Source: CAD feature listing. Evaluate the final solid. Frame: model axes, mm. A direction names the side the tool comes from. Round coordinates to 2 decimals unless told otherwise and drop trailing zeros. Loops run counter-clockwise (first coordinate to the right, second up) from the corner with the lowest first, then second, coordinate; pieces in that order, holes last. Notation, with made-up numbers: M 24.25,49.5 L 48.25,49.5 A20 cw 48.25,85.5 Z; hole C 64.25,60 d6. An arc over 180 degrees is marked long. Answer as a JSON object with one key per item and string values.
from build123d import *

# Parameters (mm, degrees)
F0_W      = 76.2
F0_H      = 38.1
F1_DEPTH  = 12.7
F2_W      = 14.097
F2_H      = 38.1
F3_DEPTH  = 0.762
F4_W      = 15.113
F4_H      = 3.048
F4_W_2    = 30.226
F5_DEPTH  = 38.101
F6_R      = 9.525
F7_DEPTH  = 6.35
F8_R      = 2.7813
F9_DEPTH  = 3.303
F10_R     = 3.3782
F11_DEPTH = 12.701
F12_R     = 0.762


with BuildPart() as f1:
    # F0 (on Top) → F1 (new body)
    with BuildSketch(Plane.XY):
        with Locations((38.1, -19.05)):
            Rectangle(F0_W, F0_H)
    extrude(amount=-F1_DEPTH)

    # F2 (on face) → F3 (cut)
    with BuildSketch(Plane.XY):
        with Locations((38.1127, -19.05)):
            Rectangle(F2_W, F2_H)
    extrude(amount=-F3_DEPTH, mode=Mode.SUBTRACT)

    # F4 (on face) → F5 (cut, through all)
    with BuildSketch(Plane(origin=(0, 0, 0), x_dir=(-1, 0, 0), z_dir=(0, 1, 0))):
        with Locations((-68.6435, -11.176)):
            Rectangle(F4_W, F4_H)
        with Locations((-38.1, -11.176)):
            Rectangle(F4_W_2, F4_H)
        with Locations((-7.5565, -11.176)):
            Rectangle(F4_W, F4_H)
    extrude(amount=-F5_DEPTH, mode=Mode.SUBTRACT)

    # F6 (on face) → F7 (cut)
    with BuildSketch(Plane(origin=(0, 0, -9.652), x_dir=(1, 0, 0), z_dir=(0, 0, -1))):
        with Locations((38.1, 19.05)):
            Circle(F6_R)
    extrude(amount=-F7_DEPTH, mode=Mode.SUBTRACT)

    # F8 (on face) → F9 (cut, through all)
    with BuildSketch(Plane(origin=(0, 0, -3.302), x_dir=(1, 0, 0), z_dir=(0, 0, -1))):
        with Locations((38.1, 19.05)):
            Circle(F8_R)
    extrude(amount=-F9_DEPTH, mode=Mode.SUBTRACT)

    # F10 (on face) → F11 (cut, through all)
    with BuildSketch(Plane(origin=(0, 0, -12.7), x_dir=(1, 0, 0), z_dir=(0, 0, -1))):
        with Locations((19.05, 19.05)):
            Circle(F10_R)
        with Locations((57.15, 19.05)):
            Circle(F10_R)
    extrude(amount=-F11_DEPTH, mode=Mode.SUBTRACT)

    # F12
    f12_edges = [f1.edges().sort_by_distance(p)[0] for p in [
        (22.987, -19.05, -9.652),
        (53.213, -19.05, -9.652),
        (15.113, -19.05, -9.652),
        (61.087, -19.05, -9.652),
    ]]
    fillet(f12_edges, radius=F12_R)


solid = f1.part
Item 1: Section C-C on y = -7. Return the cut outline in (x, z), then the cut area to 3 significant figures.
Answer sheet:
{"outline": "M 0,-9.65 L 14.35,-9.65 A0.76 cw 15.11,-10.41 L 15.11,-12.7 L 22.99,-12.7 L 22.99,-10.41 A0.76 cw 23.75,-9.65 L 52.45,-9.65 A0.76 cw 53.21,-10.41 L 53.21,-12.7 L 61.09,-12.7 L 61.09,-10.41 A0.76 cw 61.85,-9.65 L 76.2,-9.65 L 76.2,0 L 45.16,0 L 45.16,-0.76 L 31.06,-0.76 L 31.06,0 L 0,0 Z", "area": "773 mm²"}
Item 2: Pull-direction query (X, two-part tool) for faces 4 (the flat face through (69, -19, -9.652)), 5 (the flat face through (22.987, -19, -12)), 6 (the flat face through (61.087, -19, -12)); classes: pulls with the +X half, pulls with the -X half, needs draft (parallel to the pull), parting line crosses it, or undercut.
Answer sheet:
{"face 4": "needs draft", "face 5": "undercut", "face 6": "pulls with the +X half"}
Item 3: Section A-A on x = 19.05. Return the cut outline in (y, z).
Answer sheet:
{"outline": "M -38.1,-12.7 L -22.43,-12.7 L -22.43,0 L -38.1,0 Z; M -15.67,-12.7 L 0,-12.7 L 0,0 L -15.67,0 Z"}
Item 4: Section B-B on z = -1.75. Return the cut outline in (x, y), then the cut area to 3 significant figures.
Answer sheet:
{"outline": "M 0,-38.1 L 76.2,-38.1 L 76.2,0 L 0,0 Z; hole C 19.05,-19.05 d6.76; hole C 38.1,-19.05 d5.56; hole C 57.15,-19.05 d6.76", "area": "2,810 mm²"}
Item 5: Line query: probe 1 along X at (y, z) = (-19, -7); probe 2 along X at (y, z) = (-19.05, -1.8); probe 3 along X at (y, z) = (-6, -10.25). Output: solid intervals per line, ascending. Write a range as from..to.
Answer sheet:
{"probe 1": "x = 0..15.67, 22.43..28.58, 47.62..53.77, 60.53..76.2", "probe 2": "x = 0..15.67, 22.43..35.32, 40.88..53.77, 60.53..76.2", "probe 3": "x = 15.1..23, 53.2..61.1"}
Item 6: Section D-D on x = 38.1. Return the cut outline in (y, z) (3 decimals), then the cut area to 3 significant figures.
Answer sheet:
{"outline": "M -38.1,-9.652 L -28.575,-9.652 L -28.575,-3.302 L -21.831,-3.302 L -21.831,-0.762 L -38.1,-0.762 Z; M -16.269,-3.302 L -9.525,-3.302 L -9.525,-9.652 L 0,-9.652 L 0,-0.762 L -16.269,-0.762 Z", "area": "204 mm²"}
Item 7: Access query for faces 1 (the flat face through (53.213, -19, -12)), 2 (the flat face through (15.113, -19, -12)), 3 (the cylindrical face through (30.541, -13.254, -6.521)). Directions: +Z, -Z, +X, -X, +Y, -Y. A direction counts if a zero-diameter tool reaches every point of the face in a straight line with its end or side. Return the directions, or none.
Answer sheet:
{"face 1": "-Z, +Y, -Y", "face 2": "-Z, -X, +Y, -Y", "face 3": "-Z"}
Item 8: Contact query for flat-ended pins moving along their axis: pin 1 Ø7 at (x, y) = (36, -27) entering from +Z; pin 2 Ø1.1 at (y, z) = (-22, -12) entering from -X; pin 3 Ø5 at (x, y) = (38.1, -19.05) entering from +Z; pin 4 Ø3 at (x, y) = (46.5, -29) entering from -Z. Output: stop coordinate, or through.
Answer sheet:
{"pin 1": "stops at z = -0.76", "pin 2": "stops at x = 15.11", "pin 3": "passes through", "pin 4": "stops at z = -9.65"}
